```python
from build123d import *

# Parameters (mm, degrees)
MODEL_R             = 14.351
MODEL_R_2           = 2.413
MODEL_R_3           = 14.2875
BOSS_EXTRUDE1_DEPTH = 6.35
CUT_EXTRUDE1_REACH  = 8.35
SKETCH35_R          = 2.4892


with BuildPart() as part:
    # Model → Boss-Extrude1 (new body)
    with BuildSketch(Plane.XY):
        with BuildLine():
            ThreePointArc((-212.899365952, 93.541257838), (-203.778989185, 101.701881024), (-191.901103209, 104.650248016))
            Line((-191.901103209, 104.650248016), (48.661197018, 104.650248016))
            ThreePointArc((48.661197018, 104.650248016), (64.032332507, 99.471232012), (73.135172194, 86.046168785))
            Line((73.135172194, 86.046168785), (86.727013732, 37.098218434))
            ThreePointArc((86.727013732, 37.098218434), (106.36258142, 15.501750179), (127.326236921, 35.811553418))
            Line((127.326236921, 35.811553418), (140.807890588, 110.809453484))
            ThreePointArc((140.807890588, 110.809453484), (138.675228362, 126.361225539), (127.809114585, 137.689660276))
            Line((127.809114585, 137.689660276), (-44.466784077, 230.040741354))
            Line((-44.466784077, 230.040741354), (-154.507929168, 289.02994873))
            Line((-154.507929168, 289.02994873), (-199.949582693, 313.389629113))
            ThreePointArc((-199.949582693, 313.389629113), (-219.402189514, 318.224062751), (-236.303247901, 307.447705012))
            Line((-236.303247901, 307.447705012), (-425.920878295, 28.83612519))
            ThreePointArc((-425.920878295, 28.83612519), (-430.307847502, 13.679090678), (-424.898106806, -1.143726181))
            Line((-424.898106806, -1.143726181), (-385.58146606, -51.20282143))
            ThreePointArc((-385.58146606, -51.20282143), (-376.71145599, -58.357541068), (-365.605974805, -60.913979882))
            Line((-365.605974805, -60.913979882), (-324.737451002, -60.913979882))
            ThreePointArc((-324.737451002, -60.913979882), (-318.798508014, -59.439796386), (-314.23831963, -55.359484793))
            Line((-314.23831963, -55.359484793), (-212.899365952, 93.541257838))
        make_face()
        with Locations((-323.775189267, -35.513979882)):
            Circle(MODEL_R, mode=Mode.SUBTRACT)
        with Locations((-399.975189267, 2.586020118)):
            Circle(MODEL_R, mode=Mode.SUBTRACT)
        with Locations((107.189078625, 23.111553418)):
            Circle(MODEL_R_2, mode=Mode.SUBTRACT)
        with Locations((94.306236921, 35.628711714)):
            Circle(MODEL_R_2, mode=Mode.SUBTRACT)
        Polygon((110.67241113, 42.161553418), (114.338585339, 35.811553418), (110.67241113, 29.461553418), (103.340062711, 29.461553418), (99.673888502, 35.811553418), (103.340062711, 42.161553418), (106.823395217, 42.161553418), align=None, mode=Mode.SUBTRACT)
        with Locations((119.706236921, 35.994395122)):
            Circle(MODEL_R_2, mode=Mode.SUBTRACT)
        with Locations((106.823395217, 48.511553418)):
            Circle(MODEL_R_2, mode=Mode.SUBTRACT)
        with Locations((-190.707148919, 138.516914683)):
            Circle(MODEL_R, mode=Mode.SUBTRACT)
        with Locations((-208.832932893, 283.437784316)):
            Circle(MODEL_R, mode=Mode.SUBTRACT)
        with Locations((-40.935516122, 193.433854171)):
            Circle(MODEL_R_3, mode=Mode.SUBTRACT)
    extrude(amount=BOSS_EXTRUDE1_DEPTH)

    # Sketch35 → Cut-Extrude1 (cut, up to next)
    with BuildSketch(Plane.XY.offset(6.35), mode=Mode.PRIVATE) as cut_extrude1_sk1:
        with Locations((-391.784122689, 50.779120634)):
            Circle(SKETCH35_R)
    cut_extrude1_tool1 = extrude(cut_extrude1_sk1.sketch, amount=-CUT_EXTRUDE1_REACH, mode=Mode.PRIVATE) & part.part
    add(cut_extrude1_tool1.solids().sort_by_distance((-391.784123, 50.779121, 6.35))[0], mode=Mode.SUBTRACT)
    # Sketch35 → Cut-Extrude1 (cut, up to next)
    with BuildSketch(Plane.XY.offset(6.35), mode=Mode.PRIVATE) as cut_extrude1_sk2:
        with Locations((-249.731485055, 259.501852308)):
            Circle(SKETCH35_R)
    cut_extrude1_tool2 = extrude(cut_extrude1_sk2.sketch, amount=-CUT_EXTRUDE1_REACH, mode=Mode.PRIVATE) & part.part
    add(cut_extrude1_tool2.solids().sort_by_distance((-249.731485, 259.501852, 6.35))[0], mode=Mode.SUBTRACT)
    # Sketch35 → Cut-Extrude1 (cut, up to next)
    with BuildSketch(Plane.XY.offset(6.35), mode=Mode.PRIVATE) as cut_extrude1_sk3:
        with Locations((-228.733222311, 245.210842485)):
            Circle(SKETCH35_R)
    cut_extrude1_tool3 = extrude(cut_extrude1_sk3.sketch, amount=-CUT_EXTRUDE1_REACH, mode=Mode.PRIVATE) & part.part
    add(cut_extrude1_tool3.solids().sort_by_distance((-228.733222, 245.210842, 6.35))[0], mode=Mode.SUBTRACT)
    # Sketch35 → Cut-Extrude1 (cut, up to next)
    with BuildSketch(Plane.XY.offset(6.35), mode=Mode.PRIVATE) as cut_extrude1_sk4:
        with Locations((-370.785859945, 36.488110812)):
            Circle(SKETCH35_R)
    cut_extrude1_tool4 = extrude(cut_extrude1_sk4.sketch, amount=-CUT_EXTRUDE1_REACH, mode=Mode.PRIVATE) & part.part
    add(cut_extrude1_tool4.solids().sort_by_distance((-370.78586, 36.488111, 6.35))[0], mode=Mode.SUBTRACT)


solid = part.part
```
Part model, mm, in its own coordinate system. A direction names the side the tool comes from. Give positions to 0.01 mm unless a question says otherwise; leave off trailing zeros. Loops run counter-clockwise (first coordinate to the right, second up) from the corner with the lowest first, then second, coordinate; pieces in that order, holes last. Notation, with made-up numbers: M -6,-21 L 46,-21 A19 ccw 46,-12 Z; hole C 32,-27.5 d3. An arc over 180 degrees is marked long. Return JSON: item names as keys, results as strings.
1) Saw through at A-A, the plane x = -35.5. List the corners of the cut face in (y, z), then the cut area to 3 significant figures.
Calculated:
{"outline": "M 104.65,0 L 180.22,0 L 180.22,6.35 L 104.65,6.35 Z; M 206.65,0 L 225.23,0 L 225.23,6.35 L 206.65,6.35 Z", "area": "598 mm2"}
2) 3-axis set-ups, long thin cutter, end or side, ignore diameter. For faces 5 (the face through (-264.278, 18.049, 3.131)), 6 (the face through (-414.312, 3.217, 3.131)): which of +Z, -Z, +X, -X, +Y, -Y reach the whole face in a straight line?
Calculated:
{"face 5": "+Z, -Z, -Y", "face 6": "+Z, -Z"}
3) Drill centre lines: line 1 (Y direction, x = -394, z = 3.75); line 2 (X direction, y = 151, z = 2.25); line 3 (Y direction, x = -191, z = 5). Where is each one in solid material? Low to high.
Calculated:
{"line 1": "y = -40.48 to -10.46, 15.63 to 49.65, 51.91 to 75.74", "line 2": "x = -342.78 to -197.79, -183.63 to 102.98", "line 3": "y = 104.65 to 124.17, 152.86 to 308.59"}
4) Flat gauge pins, fed straight in: pin 1 Ø1.5 at (x, z) = (41, 3) entering from +Y; pin 2 Ø2 at (y, z) = (251.5, 2.5) entering from -X; pin 3 Ø3 at (x, z) = (-100.5, 2.5) entering from -Y. Where does each tip first touch, or does it go through?
Calculated:
{"pin 1": "stops at y = 184.63", "pin 2": "stops at x = -275.06", "pin 3": "stops at y = 104.65"}
5) Pull direction Y, two halves, no side cores. Call faces 1 (the face through (-329.785, 170.092, 3.131)), 2 (the face through (-149, 131, 0)), 3 (the face through (-203.93, 101.62, 3.13)), 4 (the face through (-210.701, 297.667, 3.131)): released by +Y, released by -Y, zero draft, split by the parting line, or undercut.
Calculated:
{"face 1": "released by +Y", "face 2": "zero draft", "face 3": "released by -Y", "face 4": "undercut"}
6) Saw through at C-C, the plane x = 35.5. List the corners of the cut face in (y, z), then the cut area to 3 significant figures.
Calculated:
{"outline": "M 104.65,0 L 187.17,0 L 187.17,6.35 L 104.65,6.35 Z", "area": "524 mm2"}
7) Saw through at B-B, the plane z = 4.5. Count the separate pieces of the cut face and the enclosed holes in it, then the cut area to 3 significant figures.
Calculated:
{"separate pieces": "1", "enclosed holes": "14", "area": "86,600 mm2"}
